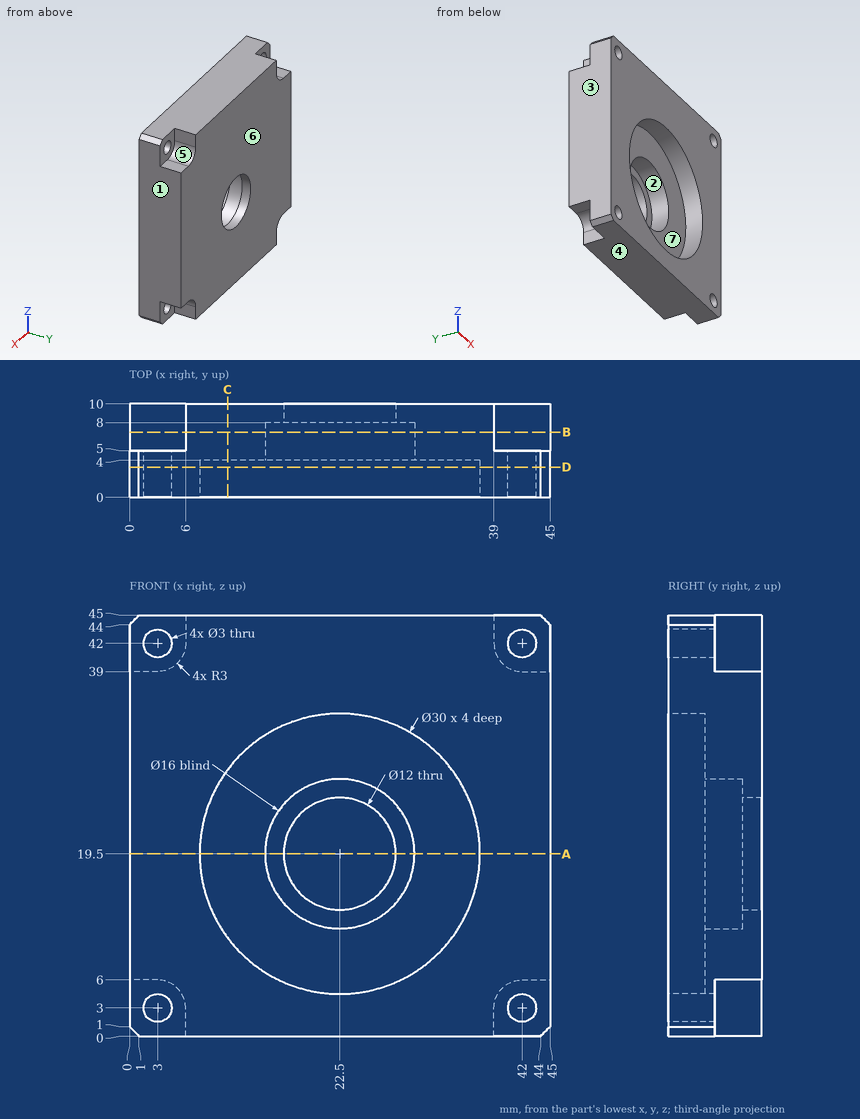
Geometry check sheet. Reference: drawing and pictorial views, mm from the part's lowest x, y, z. A direction names the side the tool comes from. Coordinates: 2 decimals unless noted, no trailing zeros. Order: outer loops, then holes, each group sorted by start corner. A loop starts at its lowest first (then second) coordinate and runs counter-clockwise, first axis right, second up.
Item 1: Tool access check on the marked faces 5, 6 and 7. Record the directions out of +Z, -Z, +X, -X, +Y, -Y that give a thin tool (end or side, any length) a straight path to the whole face; none if there is none.
Item 2: Mould release check, pull along X, two halves, no side actions. Record for the marked faces 1, 2, 3 and 4: released by +X, released by -X, zero draft, split by the parting line, or undercut.
Item 3: Scan lines: line 1 along X through (y, z) = (3, 42); line 2 along X through (y, z) = (8, 43); line 3 along Y through (x, z) = (30, 18). Record each from-to range of solid material in increasing order.
Item 4: Section check B-B (y = 7). Enter the section's corners in (x, z), plus the area to 3 significant figures.
Item 5: Section check A-A (z = 19.5). Enter the section's corners in (x, y), plus the area to 3 significant figures.
Item 6: Depth check by flat-ended pin: pin 1 (3 mm diameter, centred on x = 10.5, z = 30, fed in from -Y); pin 2 (1.5 mm diameter, centred on y = 6.5, z = 1.5, fed in from -X); pin 3 (13 mm diameter, centred on x = 20.5, z = 19, fed in from -Y); pin 4 (1.5 mm diameter, centred on x = 2, y = 8, fed in from -Z). Enter the tip coordinate at first touch or a pass-through.
Item 7: Section check C-C (x = 10.5). Enter the section's corners in (y, z), plus the area to 3 significant figures.
Item 8: Section check D-D (y = 3.25). Enter the section's corners in (x, z), plus the area to 3 significant figures.
Check sheet entries:
1. face 5: +Z, +X, +Y
1. face 6: +Z, -Z, +X, -X, +Y
1. face 7: -Y
2. face 1: released by +X
2. face 2: undercut
2. face 3: released by -X
2. face 4: zero draft
3. line 1: x = 0 to 1.5, 4.5 to 40.5, 43.5 to 45
3. line 2: x = 6 to 39
3. line 3: y = 8 to 10
4. outline: (0, 6) - (3, 6) arc R3 cw to (6, 3) - (6, 0) - (39, 0) - (39, 3) arc R3 cw to (42, 6) - (45, 6) - (45, 39) - (42, 39) arc R3 cw to (39, 42) - (39, 45) - (6, 45) - (6, 42) arc R3 cw to (3, 39) - (0, 39) - close; hole circle Ø16 at (22.5, 19.5)
4. area: 1,690 mm2
5. outline: (0, 0) - (7.5, 0) - (7.5, 4) - (14.5, 4) - (14.5, 8) - (16.5, 8) - (16.5, 10) - (0, 10) - close; (28.5, 8) - (30.5, 8) - (30.5, 4) - (37.5, 4) - (37.5, 0) - (45, 0) - (45, 10) - (28.5, 10) - close
5. area: 242 mm2
6. pin 1: stops at y = 0
6. pin 2: stops at x = 6
6. pin 3: stops at y = 4
6. pin 4: stops at z = 6
7. outline: (0, 0) - (10, 0) - (10, 45) - (0, 45) - (0, 28.5) - (4, 28.5) - (4, 10.5) - (0, 10.5) - close
7. area: 378 mm2
8. outline: (0, 1) - (1, 0) - (44, 0) - (45, 1) - (45, 44) - (44, 45) - (1, 45) - (0, 44) - close; hole circle Ø3 at (3, 3); hole circle Ø3 at (3, 42); hole circle Ø30 at (22.5, 19.5); hole circle Ø3 at (42, 3); hole circle Ø3 at (42, 42)
8. area: 1,290 mm2
